Check sheet for the drawn part. Datum: minimum x, y, z corner. Units: mm. A direction names the side the tool comes from. Round coordinates to 2 decimals unless told otherwise and drop trailing zeros. Order: outer loops, then holes, each group sorted by start corner. A loop starts at its lowest first (then second) coordinate and runs counter-clockwise, first axis right, second up. Notation, with made-up numbers: (85.25, 87.25) -> (128.25, 87.25) arc R14 cw to (128.25, 97.25) -> close; hole circle Ø8 at (72, 45.5). An arc over 180 degrees is marked (long way). Answer in a Markdown table with one row per item.
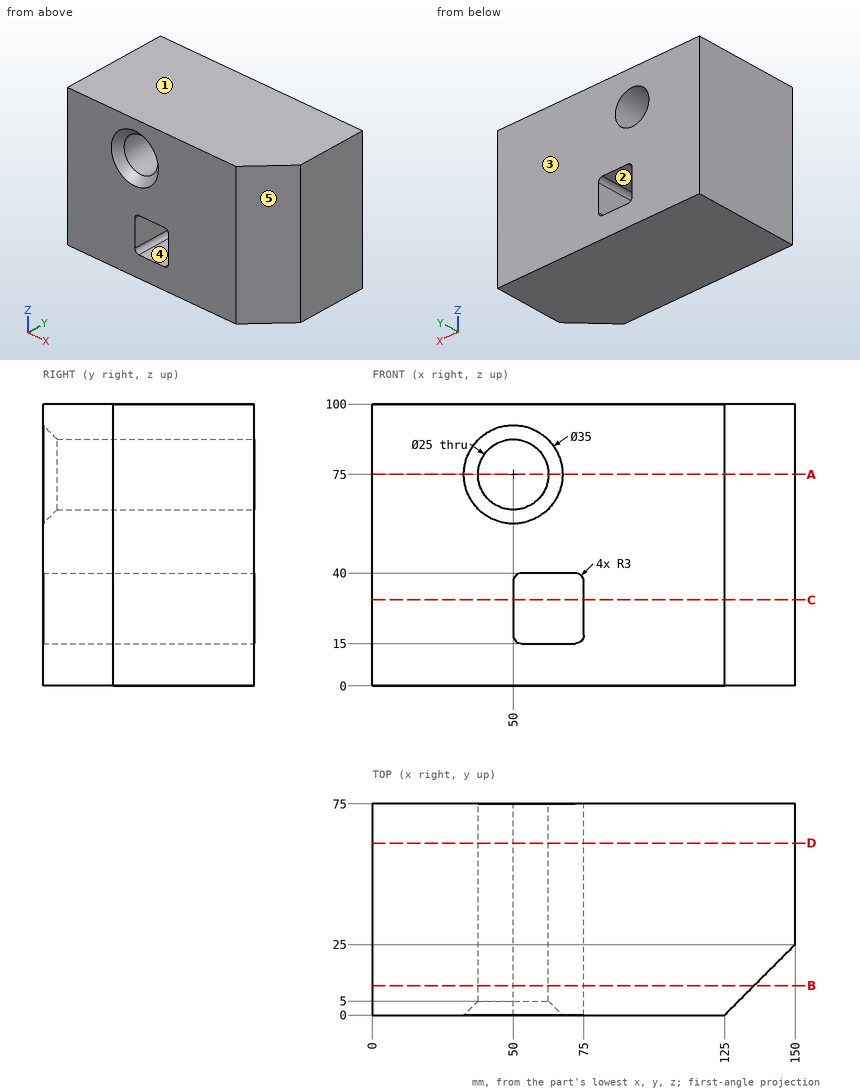
(1) Tool access check on the marked faces 1 and 2. Record the directions out of +Z, -Z, +X, -X, +Y, -Y that give a thin tool (end or side, any length) a straight path to the whole face; none if there is none.
Solutions:
| item | result |
|---|---|
| face 1 | +Z, +X, -X, +Y, -Y |
| face 2 | +Y, -Y |
(2) Section check A-A on z = 75. Record the boundary of the cut face in (x, y).
Solutions:
| item | result |
|---|---|
| outline | (0, 0) -> (32.5, 0) -> (37.5, 5) -> (37.5, 75) -> (0, 75) -> close; (62.5, 5) -> (67.5, 0) -> (125, 0) -> (150, 25) -> (150, 75) -> (62.5, 75) -> close |
(3) Section check D-D on y = 61. Record the boundary of the cut face in (x, z), plus the area to 3 significant figures.
Solutions:
| item | result |
|---|---|
| outline | (0, 0) -> (150, 0) -> (150, 100) -> (0, 100) -> close; hole circle Ø25 at (50, 75); hole (50, 18) arc R3 ccw to (53, 15) -> (72, 15) arc R3 ccw to (75, 18) -> (75, 37) arc R3 ccw to (72, 40) -> (53, 40) arc R3 ccw to (50, 37) -> close |
| area | 13,900 mm^2 |
(4) Scan lines: probe 1 along X at (y, z) = (37.5, 20); probe 2 along Z at (x, y) = (52, 24.5); probe 3 along X at (y, z) = (39, 75). Record each from-to range of solid material in increasing order. Write a range as from..to.
Solutions:
| item | result |
|---|---|
| probe 1 | 0..50, 75..150 |
| probe 2 | 0..15.17, 39.83..62.66, 87.34..100 |
| probe 3 | 0..37.5, 62.5..150 |
(5) Section check C-C on z = 30.5. Record the boundary of the cut face in (x, y), plus the area to 3 significant figures.
Solutions:
| item | result |
|---|---|
| outline | (0, 0) -> (50, 0) -> (50, 75) -> (0, 75) -> close; (75, 0) -> (125, 0) -> (150, 25) -> (150, 75) -> (75, 75) -> close |
| area | 9,060 mm^2 |
(6) Section check B-B on y = 10.5. Record the boundary of the cut face in (x, z).
Solutions:
| item | result |
|---|---|
| outline | (0, 0) -> (135.5, 0) -> (135.5, 100) -> (0, 100) -> close; hole circle Ø25 at (50, 75); hole (50, 18) arc R3 ccw to (53, 15) -> (72, 15) arc R3 ccw to (75, 18) -> (75, 37) arc R3 ccw to (72, 40) -> (53, 40) arc R3 ccw to (50, 37) -> close |
(7) Draft check along X on the marked faces 3, 4 and 5. Enter one of: pulls with the +X half, pulls with the -X half, needs draft (parallel to the pull), parting line crosses it, or undercut.
Solutions:
| item | result |
|---|---|
| face 3 | needs draft |
| face 4 | undercut |
| face 5 | pulls with the +X half |
